Geometry: see drawing. Coordinates: mm, zero at the bounding-box minimum. A direction names the side the tool comes from. Coordinates: 2 decimals unless noted, no trailing zeros. Order: outer loops, then holes, each group sorted by start corner. A loop starts at its lowest first (then second) coordinate and runs counter-clockwise, first axis right, second up.
Item 1: Section D-D on z = 2.5. Return the cut outline in (x, y).
Item 2: Section C-C on y = 26.5. Return the cut outline in (x, z), then the cut area to 3 significant figures.
Item 3: Contact query for flat-ended pins moving along their axis: P1, Ø5, axis at x = 10.5, y = 4, coming from the -Z side; P2, Ø3, axis at y = 19.5, z = 4.5, coming from the -X side. Output: stop coordinate, or through.
Item 4: Section A-A on y = 8.5. Return the cut outline in (x, z).
Item 5: Ray query, line 1 (Y direction, x = 14.5, z = 12); line 2 (Z direction, x = 16, y = 14.5); line 3 (X direction, y = 21, z = 3.5). Return the intervals inside material, ascending.
Item 6: Section B-B on x = 11.5. Return the cut outline in (y, z).
Item 7: Reachability of the marked faces 1, 2 and 3 from +Z, -Z, +X, -X, +Y, -Y: full face, straight path, thin tool, end or side. Return the list, or none.
Item 8: Mould query, pull axis Z, two halves, no side actions, for the marked faces 4, 5, 6 and 7. Classes: released by +Z, released by -Z, zero draft, split by the parting line, or undercut.
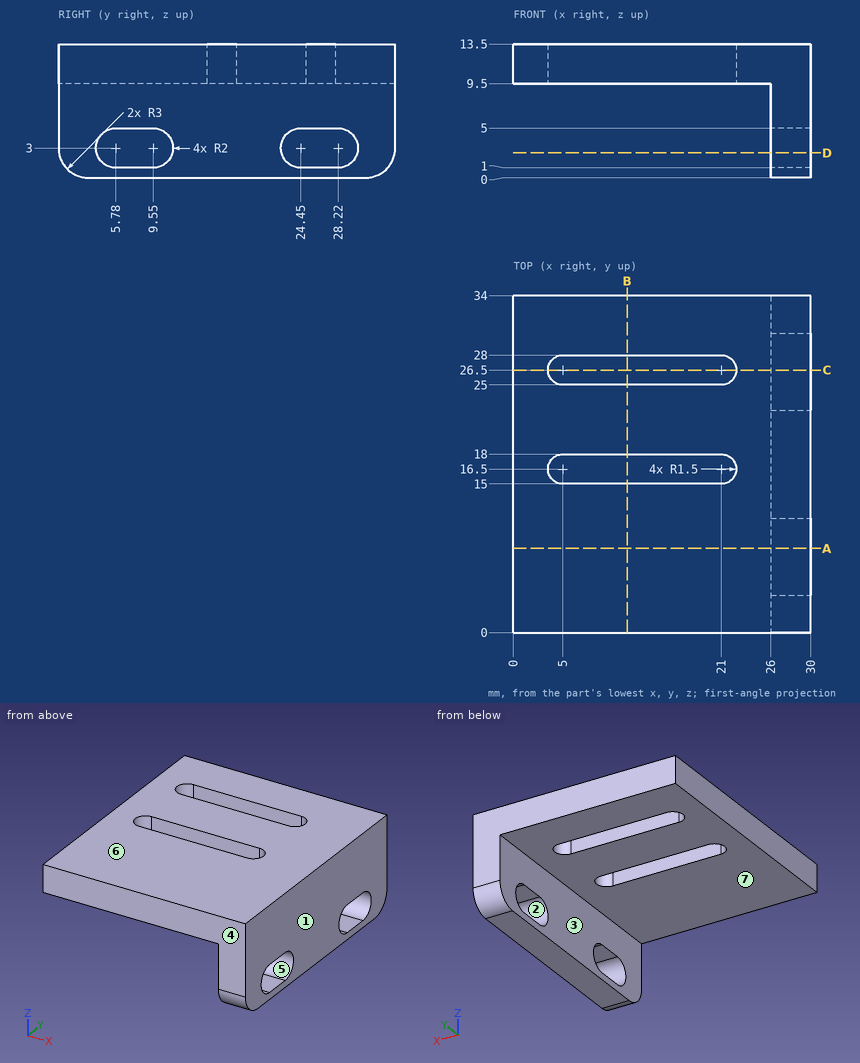
Answer list:
1. outline: (26, 0.04) - (30, 0.04) - (30, 3.84) - (26, 3.84) - close; (26, 11.49) - (30, 11.49) - (30, 22.51) - (26, 22.51) - close; (26, 30.16) - (30, 30.16) - (30, 33.96) - (26, 33.96) - close
2. outline: (0, 9.5) - (3.5, 9.5) - (3.5, 13.5) - (0, 13.5) - close; (22.5, 9.5) - (26, 9.5) - (26, 5) - (30, 5) - (30, 13.5) - (22.5, 13.5) - close; (26, 0) - (30, 0) - (30, 1) - (26, 1) - close
2. area: 66.0 mm2
3. P1: stops at z = 9.5
3. P2: stops at x = 26
4. outline: (0, 9.5) - (26, 9.5) - (26, 5) - (30, 5) - (30, 13.5) - (0, 13.5) - close; (26, 0) - (30, 0) - (30, 1) - (26, 1) - close
5. line 1: y = 0 to 15, 18 to 25, 28 to 34
5. line 2: z = 9.5 to 13.5
5. line 3: x = 26 to 30
6. outline: (0, 9.5) - (15, 9.5) - (15, 13.5) - (0, 13.5) - close; (18, 9.5) - (25, 9.5) - (25, 13.5) - (18, 13.5) - close; (28, 9.5) - (34, 9.5) - (34, 13.5) - (28, 13.5) - close
7. face 1: +Z, -Z, +X, +Y, -Y
7. face 2: +X, -X
7. face 3: -Z, -X, +Y, -Y
8. face 4: zero draft
8. face 5: undercut
8. face 6: released by +Z
8. face 7: released by -Z
